Input: part model. Units: mm. Frame: model coordinates. Give positions to 0.01 mm unless a question says otherwise; leave off trailing zeros. Loops run counter-clockwise (first coordinate to the right, second up) from the corner with the lowest first, then second, coordinate; pieces in that order, holes last. Notation, with made-up numbers: M 61.5,89 L 80.5,89 A9 ccw 80.5,99 Z; hole C 51,-35 d9. An arc over 180 degrees is marked long. One line per item, written item: value. Start each with the question number.
(1) Section A-A on x = 6. Output: boundary loops of the cut face in (y, z), plus the area to 3 significant figures.
(2) Pull-direction query (Y, two-part tool) for faces 1 (the cylindrical face through (8.54, -8.55, 9.13)), 2 (the flat face through (31, -7, 18)), 3 (the flat face through (20, 0, 9)); classes: released by +Y, released by -Y, zero draft, split by the parting line, or undercut.
(3) Section D-D on z = 5.5. Output: boundary loops of the cut face in (x, y).
(4) Pin query (flat end, axial travel): P1, Ø1, axis at x = 9.5, z = 5, coming from the +Y side. Return the tip coordinate at first contact, or that it passes through.
(5) Section C-C on z = 15.25. Output: boundary loops of the cut face in (x, y), plus the area to 3 significant figures.
(6) Ray query, line 1 along X through (y, z) = (-9.25, 3.25); line 2 along Y through (x, z) = (34, 3.75); line 3 along X through (y, z) = (-5.5, 13) (3 decimals). Return the intervals inside material, ascending. Write a range as from..to.
(7) Section B-B on y = -7.5. Output: boundary loops of the cut face in (x, z).
```python
from build123d import *

# Parameters (mm, degrees)
SKETCH_1_W          = 40
SKETCH_1_H          = 15
EXTRUDE_1_DEPTH     = 18
SKETCH_2_R          = 8
CUT_EXTRUDE_1_DEPTH = 15
SKETCH_4_R          = 2.75
CUT_EXTRUDE_2_DEPTH = 47.357307946


with BuildPart() as part:
    # 草图1 → 凸台-拉伸1 (new body)
    with BuildSketch(Plane.XY):
        with Locations((20, -7.5)):
            Rectangle(SKETCH_1_W, SKETCH_1_H)
    extrude(amount=EXTRUDE_1_DEPTH)

    # 草图2 → 切除-拉伸1 (cut)
    with BuildSketch(Plane(origin=(0, 0, 0), x_dir=(1, 0, 0), z_dir=(0, 1, 0))):
        with Locations((20, -18)):
            Circle(SKETCH_2_R)
    extrude(amount=-CUT_EXTRUDE_1_DEPTH, mode=Mode.SUBTRACT)

    # 草图4 → 切除-拉伸2 (cut, through all)
    with BuildSketch(Plane.XY.offset(18)):
        with Locations((34, -7.5)):
            Circle(SKETCH_4_R)
        with Locations((6, -7.5)):
            Circle(SKETCH_4_R)
    extrude(amount=-CUT_EXTRUDE_2_DEPTH, mode=Mode.SUBTRACT)


solid = part.part
```
Output values:
1. outline: M -15,0 L -10.25,0 L -10.25,18 L -15,18 Z; M -4.75,0 L 0,0 L 0,18 L -4.75,18 Z
1. area: 171 mm²
2. face 1: undercut
2. face 2: zero draft
2. face 3: released by +Y
3. outline: M 0,-15 L 40,-15 L 40,0 L 0,0 Z; hole C 6,-7.5 d5.5; hole C 34,-7.5 d5.5
4. P1: stops at y = 0
5. outline: M 0,-15 L 12.49,-15 L 12.49,0 L 0,0 Z; M 27.51,-15 L 40,-15 L 40,0 L 27.51,0 Z; hole C 6,-7.5 d5.5; hole C 34,-7.5 d5.5
5. area: 327 mm²
6. line 1: x = 0..3.88, 8.12..31.88, 36.12..40
6. line 2: y = -15..-10.25, -4.75..0
6. line 3: x = 0..4.113, 7.887..13.755, 26.245..32.113, 35.887..40
7. outline: M 0,0 L 3.25,0 L 3.25,18 L 0,18 Z; M 8.75,0 L 31.25,0 L 31.25,18 L 28,18 A8 cw 12,18 L 8.75,18 Z; M 36.75,0 L 40,0 L 40,18 L 36.75,18 Z
